The model under review builds one solid part; all positions refer to its coordinate system, in mm. Coordinates: 2 decimals unless noted, no trailing zeros. Write each loop counter-clockwise with the first axis right and the second up, starting at its lowest first coordinate (ties: lowest second). Pieces come first, ordered by that corner, then holes. Notation, with made-up numbers: (86.5, 7.5) - (103.5, 7.5) arc R13 ccw to (103.5, 21.5) - close; hole circle Ø2 at (77.25, 50). An arc over 180 degrees is marked (long way). Use one line per item in the form item = value. Start each with the question number.
Autodesk Inventor part; units mm, degrees
ref_plane "YZ Plane" through (0, 0, 0) normal (1, 0, 0) x (0, 1, 0)
ref_plane "XZ Plane" through (0, 0, 0) normal (0, 1, 0) x (-1, 0, 0)
ref_plane "XY Plane" through (0, 0, 0) normal (0, 0, 1) x (1, 0, 0)
sketch "スケッチ1" plane through (0, 0, 0) normal (0, 0, 1) x (1, 0, 0)
  line L0 (5, -5) -> (-5, -5)
  line L1 (-5, -5) -> (-5, 5)
  line L2 (-5, 5) -> (5, 5)
  line L3 (5, 5) -> (5, -5)
  line L4 (5, -5) -> (-5, 5) construction
  line L5 (-5, -5) -> (5, 5) construction
  point P0 (0, 0)
  dimension "d0" = 10
  dimension "d1" = 10
extrude "押し出し1" add sketch "スケッチ1" along normal blind 1
chamfer "面取り1" distance 3 distance2 1 1 edges at (0, 5, 1) measured on face at (-1.6667, 1.6667, 1)
sketch "スケッチ2" plane through (0, 0, 1) normal (0, 0, 1) x (1, 0, 0)
  circle A0 centre (-2, -2) radius 1
  circle A1 centre (2, -2) radius 1
  point P0 (0, 0)
  dimension "d7" = 2
  dimension "d8" = 2
extrude "押し出し2" cut sketch "スケッチ2" against normal blind 1
properties part number "cutter" material "アルミニウム 7075"
1. For L1, parallel to Z at x = -2.25, y = 3.75; L2, parallel to Z at x = -1, y = 4, list the stretches that pass through material, from the lowest coordinate up.
2. The part is to be moulded in two halves that separate along X. For faces 1 (the cylindrical face through (1.2, -2.6, 0.5)), 2 (the flat face through (0, 0, 0)), 3 (the flat face through (5, -1, 0.5)), 4 (the cylindrical face through (-2.8, -2.6, 0.5)), say which applies: released by +X, released by -X, zero draft, split by the parting line, or undercut.
3. Take a section at A-A (y = -2). State the section outline as (x, z) points.
4. Take a section at C-C (z = 0.45). State the section outline as (x, y) points.
Returned:
q1.L1 = 0 to 0.42
q1.L2 = 0 to 0.33
q2.face_1 = undercut
q2.face_2 = zero draft
q2.face_3 = released by +X
q2.face_4 = undercut
q3.outline = (-5, 0) - (-3, 0) - (-3, 1) - (-5, 1) - close; (-1, 0) - (1, 0) - (1, 1) - (-1, 1) - close; (3, 0) - (5, 0) - (5, 1) - (3, 1) - close
q4.outline = (-5, -5) - (5, -5) - (5, 3.65) - (-5, 3.65) - close; hole circle Ø2 at (-2, -2); hole circle Ø2 at (2, -2)
